Input: part model. Units: mm. Frame: model coordinates. Coordinates: 2 decimals unless noted, no trailing zeros. Write each loop counter-clockwise with the first axis right and the second up, starting at its lowest first coordinate (ties: lowest second). Pieces come first, ordered by that corner, then holes.
1) Section query B-B (z = 2.4). State how many separate pieces and enclosed holes the cut face has, then the cut area to 3 significant figures.
2) Section query A-A (x = -75). Output: boundary loops of the cut face in (y, z), then the cut area to 3 significant figures.
3) Pin query (flat end, axial travel): pin 1 Ø5.5 at (x, y) = (-25, 0) entering from -Z; pin 2 Ø2 at (y, z) = (-6, 1) entering from -X. Return the tip coordinate at first contact, or that it passes through.
4) Line query: L1, parallel to X at y = -3.5, z = 3.4; L2, parallel to Y at x = -75, z = 2.05; L3, parallel to X at y = 4, z = 0.75. Output: solid intervals per line, ascending.
from build123d import *

# Parameters (mm, degrees)
SKETCH1_W           = 495
SKETCH1_H           = 24
SKETCH1_R           = 4.5
BOSS_EXTRUDE1_DEPTH = 6
FILLET2_R           = 12


with BuildPart() as part:
    # Sketch1 → Boss-Extrude1 (new body)
    with BuildSketch(Plane.XY):
        Rectangle(SKETCH1_W, SKETCH1_H)
        with Locations((75, 0)):
            Circle(SKETCH1_R, mode=Mode.SUBTRACT)
        with Locations((25, 0)):
            Circle(SKETCH1_R, mode=Mode.SUBTRACT)
        with Locations((-25, 0)):
            Circle(SKETCH1_R, mode=Mode.SUBTRACT)
        with Locations((-75, 0)):
            Circle(SKETCH1_R, mode=Mode.SUBTRACT)
    extrude(amount=BOSS_EXTRUDE1_DEPTH)

    # Fillet2
    fillet2_edges = [part.edges().sort_by_distance(p)[0] for p in [
        (-247.5, -12, 3),
        (-247.5, 12, 3),
        (247.5, 12, 3),
        (247.5, -12, 3),
    ]]
    fillet(fillet2_edges, radius=FILLET2_R - 0.0001)  # a hair under: the kernel refuses the full size


solid = part.part
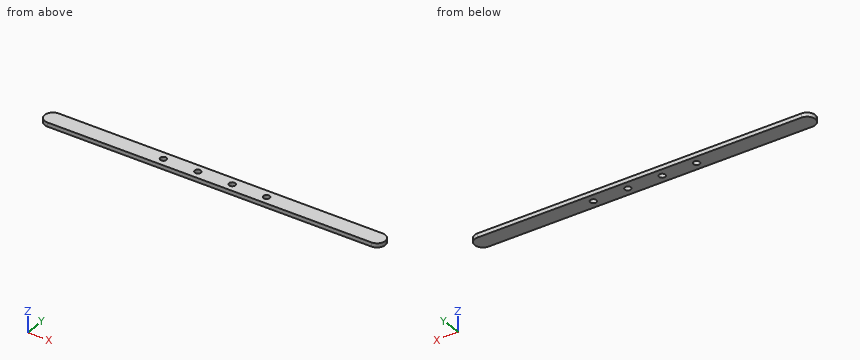
Answer:
1. separate pieces: 1
1. enclosed holes: 4
1. area: 11,500 mm2
2. outline: (-12, 0) - (-4.5, 0) - (-4.5, 6) - (-12, 6) - close; (4.5, 0) - (12, 0) - (12, 6) - (4.5, 6) - close
2. area: 90.0 mm2
3. pin 1: passes through
3. pin 2: stops at x = -246.41
4. L1: x = -246.98 to -77.83, -72.17 to -27.83, -22.17 to 22.17, 27.83 to 72.17, 77.83 to 246.98
4. L2: y = -12 to -4.5, 4.5 to 12
4. L3: x = -246.81 to -77.06, -72.94 to -27.06, -22.94 to 22.94, 27.06 to 72.94, 77.06 to 246.81
